Geometry: final body of the model. Coordinates: model frame, mm. A direction names the side the tool comes from. Round coordinates to 2 decimals unless told otherwise and drop trailing zeros. Write each loop counter-clockwise with the first axis right and the second up, starting at its lowest first coordinate (ties: lowest second). Pieces come first, ordered by that corner, then holes.
from build123d import *

# Parameters (mm, degrees)
SKETCH1_W           = 50
SKETCH1_H           = 70
SKETCH1_R           = 14
SKETCH1_R_2         = 2
SKETCH1_R_3         = 2.25
BOSS_EXTRUDE1_DEPTH = 22
M4_TAPPED_HOLE1_D   = 3.3
CHAMFER1_SIZE       = 0.5


with BuildPart() as part:
    # Sketch1 → Boss-Extrude1 (new body)
    with BuildSketch(Plane.XY):
        with Locations((5.278422274, -20.544056224)):
            Rectangle(SKETCH1_W, SKETCH1_H)
        with Locations((5.278422274, -20.544056224)):
            Circle(SKETCH1_R, mode=Mode.SUBTRACT)
        with Locations((-12.829698376, -0.544056224)):
            Circle(SKETCH1_R_2, mode=Mode.SUBTRACT)
        with Locations((-5.813457077, -0.544056224)):
            Circle(SKETCH1_R_3, mode=Mode.SUBTRACT)
        with Locations((-5.813457077, -40.544056224)):
            Circle(SKETCH1_R_3, mode=Mode.SUBTRACT)
        with Locations((-12.829698376, -40.544056224)):
            Circle(SKETCH1_R_2, mode=Mode.SUBTRACT)
        with Locations((23.386542923, -40.544056224)):
            Circle(SKETCH1_R_2, mode=Mode.SUBTRACT)
        with Locations((16.370301624, -40.544056224)):
            Circle(SKETCH1_R_3, mode=Mode.SUBTRACT)
        with Locations((16.370301624, -0.544056224)):
            Circle(SKETCH1_R_3, mode=Mode.SUBTRACT)
        with BuildLine():
            Line((22.115366155, 0.455943776), (22.115366155, -1.544056224))
            ThreePointArc((22.115366155, -1.544056224), (23.386542923, -2.815232993), (24.657719692, -1.544056224))
            Line((24.657719692, -1.544056224), (24.657719692, 0.455943776))
            ThreePointArc((24.657719692, 0.455943776), (23.386542923, 1.727120544), (22.115366155, 0.455943776))
        make_face(mode=Mode.SUBTRACT)
    extrude(amount=BOSS_EXTRUDE1_DEPTH)

    # M4 Tapped Hole1 (through all)
    with Locations(Plane.XY.offset(22)):
        with Locations((5.278422274, -0.544056224), (5.278422274, -40.544056224)):
            Hole(M4_TAPPED_HOLE1_D / 2)

    # Chamfer1
    chamfer1_edges = [part.edges().sort_by_distance(p)[0] for p in [
        (-19.721577726, 14.455943776, 11),
        (30.278422274, 14.455943776, 11),
        (30.278422274, -55.544056224, 11),
        (-19.721577726, -55.544056224, 11),
    ]]
    chamfer(chamfer1_edges, length=CHAMFER1_SIZE)


solid = part.part
1) Section A-A on x = 12. Output: boundary loops of the cut face in (y, z), plus the area to 4 significant figures.
2) Section D-D on x = -13.5. Output: boundary loops of the cut face in (y, z).
3) Section C-C on z = 1.75. State how many separate pieces and enclosed holes the cut face has, plus the area to 3 significant figures.
4) First-contact query: P1, Ø4, axis at x = 5.28, y = -0.54, coming from the -Z side; P2, Ø2.5, axis at x = 5.28, y = -40.54, coming from the +Z side. Flat tips, straight axial feed; report the tip coordinate or a pass-through.
5) Section B-B on y = -31. Output: boundary loops of the cut face in (x, z).
6) Draft query along X for faces 3 (the cylindrical face through (23.359, -2.815, 10.846)), 4 (the flat face through (-19.722, -21, 11)), 5 (the flat face through (30.278, -21, 11)). Return one class per face: pulls with the +X half, pulls with the -X half, needs draft (parallel to the pull), parting line crosses it, or undercut.
7) Reachability of faces 1 (the flat face through (22.115, -1, 11)), 2 (the flat face through (5, -55.544, 11)) from +Z, -Z, +X, -X, +Y, -Y: full face, straight path, thin tool, end or side. Return the list, or none.
8) Line query: probe 1 along X at (y, z) = (0, 16); probe 2 along Y at (x, z) = (-11.5, 9.25); probe 3 along X at (y, z) = (-0.5, 16.25). Output: solid intervals per line, ascending.
Filled in:
1. outline: (-55.54, 0) - (-32.82, 0) - (-32.82, 22) - (-55.54, 22) - close; (-8.26, 0) - (14.46, 0) - (14.46, 22) - (-8.26, 22) - close
1. area: 1,000 mm2
2. outline: (-55.54, 0) - (-42.43, 0) - (-42.43, 22) - (-55.54, 22) - close; (-38.66, 0) - (-2.43, 0) - (-2.43, 22) - (-38.66, 22) - close; (1.34, 0) - (14.46, 0) - (14.46, 22) - (1.34, 22) - close
3. separate pieces: 1
3. enclosed holes: 11
3. area: 2,760 mm2
4. P1: stops at z = 0
4. P2: passes through
5. outline: (-19.72, 0) - (-4.03, 0) - (-4.03, 22) - (-19.72, 22) - close; (14.59, 0) - (30.28, 0) - (30.28, 22) - (14.59, 22) - close
6. face 3: undercut
6. face 4: pulls with the -X half
6. face 5: pulls with the +X half
7. face 1: +Z, -Z
7. face 2: +Z, -Z, +X, -X, -Y
8. probe 1: x = -19.72 to -14.75, -10.91 to -8, -3.63 to 3.72, 6.84 to 14.19, 18.55 to 22.12, 24.66 to 30.28
8. probe 2: y = -55.54 to -42.04, -39.05 to -2.04, 0.95 to 14.46
8. probe 3: x = -19.72 to -14.83, -10.83 to -8.06, -3.56 to 3.63, 6.93 to 14.12, 18.62 to 22.12, 24.66 to 30.28
